Read the model definition and answer for the solid it produces. Units are mm, in the model's axes. A direction names the side the tool comes from. Round coordinates to 2 decimals unless told otherwise and drop trailing zeros. Write each loop counter-clockwise with the first axis right and the second up, starting at its lowest first coordinate (ties: lowest second). Pieces come first, ordered by that corner, then holes. Notation, with made-up numbers: (51.25, 23) - (72.25, 23) arc R26 cw to (72.25, 38) - close; hole circle Ø7 at (60, 12.5). An arc over 180 degrees is marked (long way). Answer as CSV lines item,"result". Start each with the question number.
1) Find section B-B on z = 29.5. Determine the outline of the cut face in (x, y), then the cut area to 3 significant figures.
2) Each of these flat-tipped pins is pushed along its axis until it touches: pin 1 (24 mm diameter, centred on y = 75.5, z = 17.5, fed in from +X); pin 2 (24 mm diameter, centred on x = -6, z = 31, fed in from +Y); pin 3 (3 mm diameter, centred on x = 0, y = 80, fed in from +Z); pin 4 (6 mm diameter, centred on y = 68.5, z = 11, fed in from -X). Where does it stop, or does it pass through?
3) Consider line 1 along Y through (x, z) = (0, 3.25); line 2 along Z through (x, y) = (0, 17.75); line 3 along X through (y, z) = (36.5, 17.5). Determine where each line is inside the solid, lowest interval first.
4) Which of the six approach directions +Z, -Z, +X, -X, +Y, -Y give full straight-line access (tool end or side, diameter ignored) to faces 5 (the flat face through (0, 65, 10)), 6 (the cylindrical face through (-32.95, 50.55, 38.04)), 7 (the cylindrical face through (-0.33, 14.79, 19.05))?
5) Find section A-A on x = 0. Determine the outline of the cut face in (y, z).
6) For a pull along X with two mould halves and no side action, classify faces 1 (the flat face through (-20, 65, 25)), 2 (the flat face through (0, 100, 25)), 3 (the flat face through (-1, 0, 20)), 4 (the flat face through (-34.857, 52.192, 16.339)) as +X half, -X half, draft (parallel to the pull), parting line (faces both ways), or undercut.
Autodesk Inventor part; units mm, degrees
ref_plane "YZ Plane" through (0, 0, 0) normal (1, 0, 0) x (0, 1, 0)
ref_plane "XZ Plane" through (0, 0, 0) normal (0, 1, 0) x (-1, 0, 0)
ref_plane "XY Plane" through (0, 0, 0) normal (0, 0, 1) x (1, 0, 0)
sketch "Sketch1" plane through (0, 0, 0) normal (0, 0, 1) x (1, 0, 0)
  arc A0 (29.8554, 102.9422) -> (-29.8554, 102.9422) centre (0, 100) ccw
  line L0 (-29.8554, 102.9422) -> (-40, 0)
  line L1 (-40, 0) -> (40, 0)
  line L2 (40, 0) -> (29.8554, 102.9422)
  point P0 (0, 0)
  point P1 (0, 0)
  dimension "d0" = 80
  dimension "d1" = 60
  dimension "d2" = 100
extrude "Extrusion1" add sketch "Sketch1" along normal blind 40
sketch "Sketch2" plane through (0, 0, 40) normal (0, 0, 1) x (1, 0, 0)
  line L0 (-20, 100) -> (20, 100)
  line L1 (20, 100) -> (20, 30)
  line L2 (20, 30) -> (-20, 30)
  line L3 (-20, 30) -> (-20, 100)
  line L4 (-40, 0) -> (40, 0)
  arc A0 (29.8554, 102.9422) -> (-29.8554, 102.9422) centre (0, 100) ccw
  point P0 (0, 0)
  point P1 (0, 100)
  point P2 (0, 0)
  point P3 (0, 130)
  dimension "d5" = 70
  dimension "d6" = 40
  dimension "d7" = 30
extrude "Extrusion2" cut sketch "Sketch2" against normal blind 30
fillet "Fillet1" radius 6.858 3 edges at (0, 130, 40) (-34.9277, 51.4711, 40) (34.9277, 51.4711, 40)
sketch "Sketch3" plane through (-40, 0, 0) normal (0, -1, 0) x (1, 0, 0)
  line L0 (0, 0) -> (80, 0)
  line L1 (80, 0) -> (80, 33.142)
  line L2 (6.8912, 40) -> (73.1088, 40)
  circle A0 centre (40, 16.571) radius 2.5
  point P0 (40, 0)
  point P1 (40, 40)
  point P2 (80, 16.571)
  dimension "d11" = 5
extrude "Extrusion3" cut sketch "Sketch3" against normal blind 30
sketch "Sketch4" plane through (0, 0, 10) normal (0, 0, 1) x (1, 0, 0)
  circle A0 centre (0, 80) radius 2.5
  line L0 (20, 30) -> (-20, 30)
  line L1 (20, 100) -> (20, 30)
  line L2 (-20, 100) -> (20, 100)
  line L3 (-20, 30) -> (-20, 100)
  point P0 (0, 0)
  dimension "d14" = 20
  dimension "d15" = 5
  dimension "d16" = 20
extrude "Extrusion4" cut sketch "Sketch4" against normal blind 30 contours A0
properties part number "Robot_arm_3"
Check values:
1,outline,"(-40, 0) - (40, 0) - (29.86, 102.94) arc R30 ccw to (-29.86, 102.94) - close; hole (-20, 30) - (20, 30) - (20, 100) - (-20, 100) - close"
1,area,"5,630 mm^2"
2,pin 1,"stops at x = 33.74"
2,pin 2,"stops at y = 130"
2,pin 3,"passes through"
2,pin 4,"stops at x = -33.55"
3,line 1,"y = 0 to 77.5, 82.5 to 130"
3,line 2,"z = 0 to 14.07, 19.07 to 40"
3,line 3,"x = -36.4 to -20, 20 to 36.4"
4,face 5,"+Z"
4,face 6,"+Z, -X, +Y"
4,face 7,"-Y"
5,outline,"(0, 0) - (77.5, 0) - (77.5, 10) - (30, 10) - (30, 14.07) - (0, 14.07) - close; (0, 19.07) - (30, 19.07) - (30, 40) - (0, 40) - close; (82.5, 0) - (130, 0) - (130, 33.14) arc R6.86 ccw to (123.14, 40) - (100, 40) - (100, 10) - (82.5, 10) - close"
6,face 1,"undercut"
6,face 2,"undercut"
6,face 3,"draft"
6,face 4,"-X half"
